from build123d import *

# Parameters (mm, degrees)
SKETCH1_W               = 95.25
SKETCH1_H               = 50.8
BOSS_EXTRUDE1_DEPTH     = 3
CUT_EXTRUDE1_DEPTH      = 55.058307641
CUT_EXTRUDE1_DEPTH_BACK = 55.058307641
SKETCH2_R               = 2.1
CUT_EXTRUDE3_DEPTH      = 55.058307641
CUT_EXTRUDE3_DEPTH_BACK = 55.058307641
SKETCH4_R               = 7.5
CUT_EXTRUDE4_DEPTH      = 55.058307641
CUT_EXTRUDE4_DEPTH_BACK = 55.058307641
SKETCH5_W               = 24.95556865
SKETCH5_H               = 50.8


with BuildPart() as part:
    # Sketch1 → Boss-Extrude1 (new body)
    with BuildSketch(Plane(origin=(0, 0, 0), x_dir=(1, 0, 0), z_dir=(0, 1, 0))):
        Rectangle(SKETCH1_W, SKETCH1_H)
    extrude(amount=BOSS_EXTRUDE1_DEPTH)

    # Sketch2 → Cut-Extrude1 (cut, two sides: drawn at the far end of the back side and taken through both)
    with BuildSketch(Plane(origin=(0, 3, 0), x_dir=(1, 0, 0), z_dir=(0, 1, 0)).offset(-CUT_EXTRUDE1_DEPTH_BACK)):
        with Locations(Location((-17.68, 17.68, 0), (0, 0, 270))):
            Circle(SKETCH2_R)
        with Locations(Location((17.68, 17.68, 0), (0, 0, 270))):
            Circle(SKETCH2_R)
        with Locations(Location((17.68, -17.68, 0), (0, 0, 270))):
            Circle(SKETCH2_R)
        with Locations(Location((-17.68, -17.68, 0), (0, 0, 270))):
            Circle(SKETCH2_R)
    extrude(amount=CUT_EXTRUDE1_DEPTH + CUT_EXTRUDE1_DEPTH_BACK, mode=Mode.SUBTRACT)

    # Sketch4 → Cut-Extrude3 (cut, two sides: drawn at the far end of the back side and taken through both)
    with BuildSketch(Plane(origin=(0, 3, 0), x_dir=(1, 0, 0), z_dir=(0, 1, 0)).offset(-CUT_EXTRUDE3_DEPTH_BACK)):
        with Locations(Location((0, 0, 0), (0, 0, 270))):
            Circle(SKETCH4_R)
    extrude(amount=CUT_EXTRUDE3_DEPTH + CUT_EXTRUDE3_DEPTH_BACK, mode=Mode.SUBTRACT)

    # Sketch5 → Cut-Extrude4 (cut, two sides: drawn at the far end of the back side and taken through both)
    with BuildSketch(Plane(origin=(0, 3, 0), x_dir=(1, 0, 0), z_dir=(0, 1, 0)).offset(-CUT_EXTRUDE4_DEPTH_BACK)):
        with Locations((35.147215675, 0)):
            Rectangle(SKETCH5_W, SKETCH5_H)
    extrude(amount=CUT_EXTRUDE4_DEPTH + CUT_EXTRUDE4_DEPTH_BACK, mode=Mode.SUBTRACT)


solid = part.part
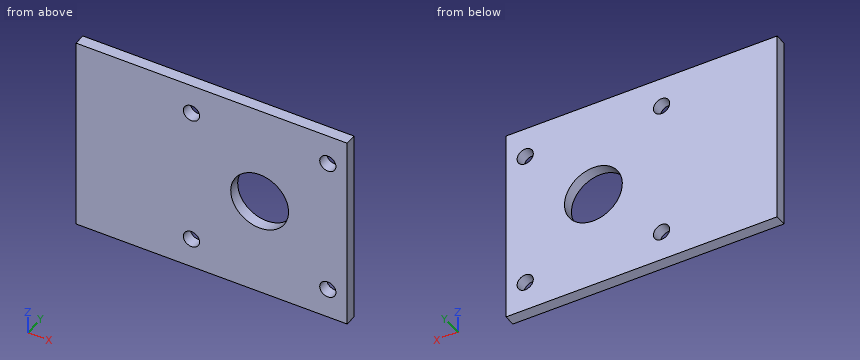
Check sheet for the modelled part. Datum: model origin and axes. Units: mm. Round coordinates to 2 decimals unless told otherwise and drop trailing zeros. Order: outer loops, then holes, each group sorted by start corner. A loop starts at its lowest first (then second) coordinate and runs counter-clockwise, first axis right, second up. Notation, with made-up numbers: M 38,44.5 L 57,44.5 A29 cw 57,80.5 Z; hole C 25,65.25 d1. An arc over 180 degrees is marked long. One line per item, written item: value. Start each with the question number.
1. Section check C-C on y = 2. Enter the section's corners in (x, z) (3 decimals).
2. Section check A-A on x = 0. Enter the section's corners in (y, z), and give its area (3 significant figures).
3. Scan lines: line 1 along X through (y, z) = (1.7, -17.68) (3 decimals); line 2 along Z through (x, y) = (-17.68, 0.65); line 3 along X through (y, z) = (1.1, 0) (3 decimals). Record each from-to range of solid material in increasing order.
4. Section check D-D on x = -17.68. Enter the section's corners in (y, z).
5. Gauge pin test, flat end, axial feed: P1, Ø3.5, axis at x = -17.68, z = -17.68, coming from the -Y side. Record the tip position at first contact, or that the pin passes through.
6. Section check B-B on z = 0. Enter the section's corners in (x, y) (3 decimals), and give its area (3 significant figures).
Results found:
1. outline: M -47.625,-25.4 L 22.669,-25.4 L 22.669,25.4 L -47.625,25.4 Z; hole C -17.68,-17.68 d4.2; hole C -17.68,17.68 d4.2; hole C 0,0 d15; hole C 17.68,-17.68 d4.2; hole C 17.68,17.68 d4.2
2. outline: M 0,-25.4 L 3,-25.4 L 3,-7.5 L 0,-7.5 Z; M 0,7.5 L 3,7.5 L 3,25.4 L 0,25.4 Z
2. area: 107 mm^2
3. line 1: -47.625 to -19.78, -15.58 to 15.58, 19.78 to 22.669
3. line 2: -25.4 to -19.78, -15.58 to 15.58, 19.78 to 25.4
3. line 3: -47.625 to -7.5, 7.5 to 22.669
4. outline: M 0,-25.4 L 3,-25.4 L 3,-19.78 L 0,-19.78 Z; M 0,-15.58 L 3,-15.58 L 3,15.58 L 0,15.58 Z; M 0,19.78 L 3,19.78 L 3,25.4 L 0,25.4 Z
5. P1: through
6. outline: M -47.625,0 L -7.5,0 L -7.5,3 L -47.625,3 Z; M 7.5,0 L 22.669,0 L 22.669,3 L 7.5,3 Z
6. area: 166 mm^2
